The model under review builds one solid part; all positions refer to its coordinate system, in mm. A direction names the side the tool comes from. Round coordinates to 2 decimals unless told otherwise and drop trailing zeros. Loops run counter-clockwise (first coordinate to the right, second up) from the corner with the lowest first, then second, coordinate; pieces in that order, holes last. Notation, with made-up numbers: M 63.25,-26.5 L 96.25,-26.5 A11 ccw 96.25,-18.5 Z; hole C 41,88.25 d11. An arc over 180 degrees is marked long. Answer as a JSON object with one key per item and string values. Group by question number.
Item 1: The part is to be moulded in two halves that separate along Y. For faces 3 (the face through (-5.822, 1.533, 0.789)), 4 (the face through (0, 11.912, 1)), 5 (the face through (0, -11.912, 1)), say which applies: +Y half, -Y half, draft (parallel to the pull), parting line (faces both ways), or undercut.
Item 2: Insertion check: P1, Ø0.7, axis at x = 6.35, y = 9.37, coming from the +Z side; P2, Ø3, axis at x = 2.5, y = -3.5, coming from the -Z side. Each pin has a flat end and moves straight along its axis. Give the tip position at first contact, or say it passes through.
Item 3: Consider section C-C (z = 1.1). State how many separate pieces and enclosed holes the cut face has, and give its area (3 significant figures).
Item 4: Consider section B-B (x = 2.5). Give the boundary of the cut face in (y, z).
Item 5: Consider section D-D (x = -2.75). Give the boundary of the cut face in (y, z), and give its area (3 significant figures).
Item 6: Tool access review of faces 1 (the face through (-6, -2.407, 1)), 2 (the face through (-7.62, 0, 1)): name each direction out of +Z, -Z, +X, -X, +Y, -Y from which nothing blocks a thin tool from reaching the whole face with its end or side.
Item 7: Consider section A-A (x = -6.35). Give the boundary of the cut face in (y, z), and give its area (3 significant figures).
Item 8: To check wall thickness, follow line 1 (Y direction, x = -2.5, z = 0.85); line 2 (X direction, y = 7.25, z = 0.95); line 3 (Y direction, x = -5.25, z = 0.9). State the ranges of each line that lie inside material, in increasing order.
```python
from build123d import *

# Parameters (mm, degrees)
F0_W     = 15.24
F0_H     = 23.82343
F0_R     = 0.5715
F1_DEPTH = 1.6
F2_R     = 0.5
F2_W     = 1.8034
F2_H     = 2.5908
F3_DEPTH = 1.601


with BuildPart() as f1:
    # F0 (on Top) → F1 (new body)
    with BuildSketch(Plane.XY):
        Rectangle(F0_W, F0_H)
        with Locations((-6.35, -0.788285)):
            Circle(F0_R, mode=Mode.SUBTRACT)
        with Locations((6.35, -0.788285)):
            Circle(F0_R, mode=Mode.SUBTRACT)
        with Locations((-6.35, 1.751715)):
            Circle(F0_R, mode=Mode.SUBTRACT)
        with Locations((-6.35, 4.291715)):
            Circle(F0_R, mode=Mode.SUBTRACT)
        with Locations((-6.35, 6.831715)):
            Circle(F0_R, mode=Mode.SUBTRACT)
        with Locations((-6.35, 9.371715)):
            Circle(F0_R, mode=Mode.SUBTRACT)
        with Locations((6.35, 1.751715)):
            Circle(F0_R, mode=Mode.SUBTRACT)
        with Locations((6.35, 4.291715)):
            Circle(F0_R, mode=Mode.SUBTRACT)
        with Locations((6.35, 6.831715)):
            Circle(F0_R, mode=Mode.SUBTRACT)
        with Locations((6.35, 9.371715)):
            Circle(F0_R, mode=Mode.SUBTRACT)
    extrude(amount=F1_DEPTH)

    # F2 (on Top) → F3 (cut, through all)
    with BuildSketch(Plane.XY):
        with Locations((2.5019, -10.712373)):
            Circle(F2_R)
        with Locations((0, 3.791027)):
            Circle(F2_R)
        with Locations((-2.5, 3.791027)):
            Circle(F2_R)
        with Locations((-2.5019, -10.712373)):
            Circle(F2_R)
        with Locations((2.5, 3.791027)):
            Circle(F2_R)
        with Locations((-5.7023, -3.701973)):
            Rectangle(F2_W, F2_H)
        with Locations((5.7023, -3.701973)):
            Rectangle(F2_W, F2_H)
    extrude(amount=F3_DEPTH, mode=Mode.SUBTRACT)


solid = f1.part
```
Geometry results:
{
 "1": {"face 3": "undercut", "face 4": "+Y half", "face 5": "-Y half"},
 "2": {"P1": "passes through", "P2": "stops at z = 0"},
 "3": {"separate pieces": "1", "enclosed holes": "17", "area": "340 mm^2"},
 "4": {"outline": "M -11.91,0 L -11.21,0 L -11.21,1.6 L -11.91,1.6 Z; M -10.21,0 L 3.29,0 L 3.29,1.6 L -10.21,1.6 Z; M 4.29,0 L 11.91,0 L 11.91,1.6 L 4.29,1.6 Z"},
 "5": {"outline": "M -11.91,0 L -11.15,0 L -11.15,1.6 L -11.91,1.6 Z; M -10.28,0 L 3.36,0 L 3.36,1.6 L -10.28,1.6 Z; M 4.22,0 L 11.91,0 L 11.91,1.6 L 4.22,1.6 Z", "area": "35.3 mm^2"},
 "6": {"face 1": "+Z, -Z", "face 2": "+Z, -Z, -X, +Y, -Y"},
 "7": {"outline": "M -11.91,0 L -5,0 L -5,1.6 L -11.91,1.6 Z; M -2.41,0 L -1.36,0 L -1.36,1.6 L -2.41,1.6 Z; M -0.22,0 L 1.18,0 L 1.18,1.6 L -0.22,1.6 Z; M 2.32,0 L 3.72,0 L 3.72,1.6 L 2.32,1.6 Z; M 4.86,0 L 6.26,0 L 6.26,1.6 L 4.86,1.6 Z; M 7.4,0 L 8.8,0 L 8.8,1.6 L 7.4,1.6 Z; M 9.94,0 L 11.91,0 L 11.91,1.6 L 9.94,1.6 Z", "area": "24.8 mm^2"},
 "8": {"line 1": "y = -11.91 to -11.21, -10.21 to 3.29, 4.29 to 11.91", "line 2": "x = -7.62 to -6.74, -5.96 to 5.96, 6.74 to 7.62", "line 3": "y = -11.91 to -5, -2.41 to 11.91"}
}
